from build123d import *

# Parameters (mm, degrees)
F0_W     = 1524
F0_H     = 762
F1_DEPTH = 381
F2_R     = 101.6
F3_W     = 914.4
F3_H     = 457.2
F4_DEPTH = 254
F5_R     = 101.6
F6_R     = 19.05
F7_DEPTH = 381.001
F8_R     = 19.05
F9_DEPTH = 381.001


with BuildPart() as f1:
    # F0 (on Top) → F1 (new body)
    with BuildSketch(Plane.XY):
        Rectangle(F0_W, F0_H)
    extrude(amount=F1_DEPTH)

    # F2
    f2_edges = [f1.edges().sort_by_distance(p)[0] for p in [
        (-762, 381, 190.5),
        (-762, -381, 190.5),
        (762, -381, 190.5),
        (762, 381, 190.5),
    ]]
    fillet(f2_edges, radius=F2_R)

    # F3 (on face) → F4 (cut)
    with BuildSketch(Plane.XY.offset(381)):
        with Locations((0, -25.4)):
            Rectangle(F3_W, F3_H)
    extrude(amount=-F4_DEPTH, mode=Mode.SUBTRACT)

    # F5
    f5_edges = [f1.edges().sort_by_distance(p)[0] for p in [
        (-457.2, 203.2, 254),
        (457.2, 203.2, 254),
        (457.2, -254, 254),
        (-457.2, -254, 254),
        (-457.2, -25.4, 127),
        (0, -254, 127),
        (457.2, -25.4, 127),
        (0, 203.2, 127),
    ]]
    fillet(f5_edges, radius=F5_R)

    # F6 (on face) → F7 (cut, through all)
    with BuildSketch(Plane.XY.offset(381)):
        with Locations((-76.2, 292.1)):
            Circle(F6_R)
    extrude(amount=-F7_DEPTH, mode=Mode.SUBTRACT)

    # F8 (on face) → F9 (cut, through all)
    with BuildSketch(Plane.XY.offset(381)):
        with Locations((76.2, 292.1)):
            Circle(F8_R)
    extrude(amount=-F9_DEPTH, mode=Mode.SUBTRACT)


solid = f1.part
Design review of the part built by this model. Coordinates are the model's own, in mm. A direction names the side the tool comes from. Round coordinates to 2 decimals unless told otherwise and drop trailing zeros. Write each loop counter-clockwise with the first axis right and the second up, starting at its lowest first coordinate (ties: lowest second). Pieces come first, ordered by that corner, then holes. Notation, with made-up numbers: (-22.75, 7.5) - (21.25, 7.5) arc R12 cw to (21.25, 20.5) - close; hole circle Ø7 at (30.5, 69). An arc over 180 degrees is marked (long way). Use a Markdown table: item, result. Add a question column.
1. For faces 1 (the face through (-80.33, 273.503, 193.167)), 2 (the face through (426.648, -225.028, 303.733)), list the 3-axis set-ups (+Z, -Z, +X, -X, +Y, -Y) from which the entire face can be reached by the end or side of a thin tool; tool diameter is ignored.
2. We need section A-A (x = 76.2). State the section outline as (y, z) points.
3. Mouldability with a two-part tool opening along X and no side actions: class faces 3 (the face through (4.978, 174.228, 157.552)), 4 (the face through (731.448, -352.028, 193.167)), 5 (the face through (-11, 259, 381)) as +X half, -X half, draft (parallel to the pull), parting line (faces both ways), or undercut.
4. Wall thickness on probe 1 along Y at (x, z) = (76.2, 109); probe 2 along Y at (x, z) = (76, 219); probe 3 along Y at (x, z) = (-76.2, 164): over which ranges is each line inside the solid? List them lowest first.
5. Clearance check with flat-ended pins moving along their axes: pin 1 (10 mm diameter, centred on y = -289, z = 329, fed in from -X); pin 2 (10 mm diameter, centred on x = -204.5, y = -117.5, fed in from +Z). State where each tip first meets the part, or that it passes through.
6. We need section B-B (y = -25). State the section outline as (x, z) points.
7. We need section C-C (x = 304.5). State the section outline as (y, z) points.
8. We need section D-D (z = 189). State the section outline as (x, y) points.
Output:
| question | item | result |
|---|---|---|
| 1 | face 1 | +Z, -Z |
| 1 | face 2 | +Z |
| 2 | outline | (-381, 0) - (273.05, 0) - (273.05, 381) - (203.2, 381) - (203.2, 228.6) arc R101.6 cw to (101.6, 127) - (-152.4, 127) arc R101.6 cw to (-254, 228.6) - (-254, 381) - (-381, 381) - close; (311.15, 0) - (381, 0) - (381, 381) - (311.15, 381) - close |
| 3 | face 3 | undercut |
| 3 | face 4 | +X half |
| 3 | face 5 | draft |
| 4 | probe 1 | y = -381 to 273.05, 311.15 to 381 |
| 4 | probe 2 | y = -381 to -253.55, 202.75 to 273.05, 311.15 to 381 |
| 4 | probe 3 | y = -381 to -230.82, 180.02 to 273.05, 311.15 to 381 |
| 5 | pin 1 | stops at x = -761.9 |
| 5 | pin 2 | stops at z = 127 |
| 6 | outline | (-762, 0) - (762, 0) - (762, 381) - (457.2, 381) - (457.2, 228.6) arc R101.6 cw to (355.6, 127) - (-355.6, 127) arc R101.6 cw to (-457.2, 228.6) - (-457.2, 381) - (-762, 381) - close |
| 7 | outline | (-381, 0) - (381, 0) - (381, 381) - (203.2, 381) - (203.2, 228.6) arc R101.6 cw to (101.6, 127) - (-152.4, 127) arc R101.6 cw to (-254, 228.6) - (-254, 381) - (-381, 381) - close |
| 8 | outline | (-762, -279.4) arc R101.6 ccw to (-660.4, -381) - (660.4, -381) arc R101.6 ccw to (762, -279.4) - (762, 279.4) arc R101.6 ccw to (660.4, 381) - (-660.4, 381) arc R101.6 ccw to (-762, 279.4) - close; hole (-449.16, -152.4) arc R93.56 ccw to (-355.6, -245.96) - (355.6, -245.96) arc R93.56 ccw to (449.16, -152.4) - (449.16, 101.6) arc R93.56 ccw to (355.6, 195.16) - (-355.6, 195.16) arc R93.56 ccw to (-449.16, 101.6) - close; hole circle Ø38.1 at (-76.2, 292.1); hole circle Ø38.1 at (76.2, 292.1) |
